```python
from build123d import *

# Parameters (mm, degrees)
SKETCH1_W           = 20.7
SKETCH1_H           = 13.5
BOSS_EXTRUDE1_DEPTH = 2
FILLET1_R           = 0.5
SKETCH2_W           = 10.6
SKETCH2_H           = 3.6
SKETCH2_W_2         = 7.1
SKETCH2_H_2         = 7.1
SKETCH2_W_3         = 1.7
SKETCH2_H_3         = 4.85
CUT_EXTRUDE1_DEPTH  = 13.517387906


with BuildPart() as part:
    # Sketch1 → Boss-Extrude1 (new body)
    with BuildSketch(Plane.XY):
        Rectangle(SKETCH1_W, SKETCH1_H)
    extrude(amount=BOSS_EXTRUDE1_DEPTH)

    # Fillet1
    fillet1_edges = [part.edges().sort_by_distance(p)[0] for p in [
        (-10.35, 0, 2),
        (0, -6.75, 2),
        (10.35, 0, 2),
        (0, -6.75, 0),
        (-10.35, 0, 0),
        (0, 6.75, 0),
        (10.35, 0, 0),
        (10.35, -6.75, 1),
        (-10.35, -6.75, 1),
        (-10.35, 6.75, 1),
        (10.35, 6.75, 1),
        (0, 6.75, 2),
    ]]
    fillet(fillet1_edges, radius=FILLET1_R)

    # Sketch2 → Cut-Extrude1 (cut, through all)
    with BuildSketch(Plane.XY.offset(2)):
        Rectangle(SKETCH2_W, SKETCH2_H)
        Rectangle(SKETCH2_W_2, SKETCH2_H_2)
        with Locations((0, 2.425)):
            Rectangle(SKETCH2_W_3, SKETCH2_H_3)
    extrude(amount=-CUT_EXTRUDE1_DEPTH, mode=Mode.SUBTRACT)


solid = part.part
```
Here's how the part is built. I have some questions about the finished solid (model axes, mm). A direction names the side the tool comes from. Give positions to 0.01 mm unless a question says otherwise; leave off trailing zeros. Order: outer loops, then holes, each group sorted by start corner. A loop starts at its lowest first (then second) coordinate and runs counter-clockwise, first axis right, second up. Notation, with made-up numbers: (-16.5, 84.25) - (21.5, 84.25) arc R13 cw to (21.5, 92.25) - close; hole circle Ø7 at (34, 33.5). An arc over 180 degrees is marked (long way). Answer as a JSON object with one key per item and string values. Group by question number.
Item 1: If we section it at B-B on x = 0.5: Please give me the cut outline in (y, z).
Item 2: If we section it at C-C on z = 0.85: Please give me the cut outline in (x, y), and give its area (3 significant figures).
Item 3: If we section it at A-A on y = 0.25: Please give me the cut outline in (x, z).
Item 4: Which directions (+Z, -Z, +X, -X, +Y, -Y) give clear straight access to the entire face, cutting with the end or side of a thin tool? Please do faces 4 (the flat face through (4, -1.8, 1)), 5 (the flat face through (10.35, 0, 1)).
Item 5: Please list where these lines run through material, in increasing order: probe 1 along X at (y, z) = (-1.5, 0.65); probe 2 along Y at (x, z) = (4.5, 0.95).
Item 6: If we section it at D-D on z = 1.8: Please give me the cut outline in (x, y), and give its area (3 significant figures).
Item 7: If we mould it in two halves opening along Y, with no side actions, what happens to faces 1 (the flat face through (0, -3.55, 1)), 2 (the flat face through (0, -6.75, 1)), 3 (the flat face through (-10.35, 0, 1))? For each: pulls with the +Y half, pulls with the -Y half, needs draft (parallel to the pull), parting line crosses it, or undercut.
Result set:
{
 "1": {"outline": "(-6.75, 0.5) arc R0.5 ccw to (-6.25, 0) - (-3.55, 0) - (-3.55, 2) - (-6.25, 2) arc R0.5 ccw to (-6.75, 1.5) - close; (4.85, 0) - (6.25, 0) arc R0.5 ccw to (6.75, 0.5) - (6.75, 1.5) arc R0.5 ccw to (6.25, 2) - (4.85, 2) - close"},
 "2": {"outline": "(-10.35, -6.25) arc R0.5 ccw to (-9.85, -6.75) - (9.85, -6.75) arc R0.5 ccw to (10.35, -6.25) - (10.35, 6.25) arc R0.5 ccw to (9.85, 6.75) - (-9.85, 6.75) arc R0.5 ccw to (-10.35, 6.25) - close; hole (-5.3, -1.8) - (-3.55, -1.8) - (-3.55, -3.55) - (3.55, -3.55) - (3.55, -1.8) - (5.3, -1.8) - (5.3, 1.8) - (3.55, 1.8) - (3.55, 3.55) - (0.85, 3.55) - (0.85, 4.85) - (-0.85, 4.85) - (-0.85, 3.55) - (-3.55, 3.55) - (-3.55, 1.8) - (-5.3, 1.8) - close", "area": "214 mm²"},
 "3": {"outline": "(-10.35, 0.5) arc R0.5 ccw to (-9.85, 0) - (-5.3, 0) - (-5.3, 2) - (-9.85, 2) arc R0.5 ccw to (-10.35, 1.5) - close; (5.3, 0) - (9.85, 0) arc R0.5 ccw to (10.35, 0.5) - (10.35, 1.5) arc R0.5 ccw to (9.85, 2) - (5.3, 2) - close"},
 "4": {"face 4": "+Z, -Z", "face 5": "+Z, -Z, +X, +Y, -Y"},
 "5": {"probe 1": "-10.35 to -5.3, 5.3 to 10.35", "probe 2": "-6.75 to -1.8, 1.8 to 6.75"},
 "6": {"outline": "(-10.25, -6.25) arc R0.4 ccw to (-9.85, -6.65) - (9.85, -6.65) arc R0.4 ccw to (10.25, -6.25) - (10.25, 6.25) arc R0.4 ccw to (9.85, 6.65) - (-9.85, 6.65) arc R0.4 ccw to (-10.25, 6.25) - close; hole (-5.3, -1.8) - (-3.55, -1.8) - (-3.55, -3.55) - (3.55, -3.55) - (3.55, -1.8) - (5.3, -1.8) - (5.3, 1.8) - (3.55, 1.8) - (3.55, 3.55) - (0.85, 3.55) - (0.85, 4.85) - (-0.85, 4.85) - (-0.85, 3.55) - (-3.55, 3.55) - (-3.55, 1.8) - (-5.3, 1.8) - close", "area": "207 mm²"},
 "7": {"face 1": "undercut", "face 2": "pulls with the -Y half", "face 3": "needs draft"}
}
